Can you work these out from the model? Positions are in its coordinate system, mm. Give positions to 0.01 mm unless a question says otherwise; leave off trailing zeros. Loops run counter-clockwise (first coordinate to the right, second up) from the corner with the lowest first, then second, coordinate; pieces in that order, holes last. Notation, with made-up numbers: (53.25, 10.5) - (86.25, 10.5) arc R22 cw to (86.25, 35.5) - close; hole circle Ø6 at (-12.5, 45.25). An arc over 180 degrees is marked (long way). Answer in a Markdown table with one row per item.
from build123d import *

# Parameters (mm, degrees)
BOSS_EXTRUDE1_DEPTH = 0.05
FILLET1_R           = 1


with BuildPart() as part:
    # frame_outline → Boss-Extrude1 (new, symmetric)
    with BuildSketch(Plane.XY):
        Polygon((0, 0), (3, 0), (3, -0.25), (4, -0.25), (4, 0), (4.5, 0), (5.266044443, 0.64278761), (5.426741346, 0.451276499), (6.192785789, 1.094064109), (6.032088886, 1.285575219), (6.606622219, 1.767665927), (5.050898392, 1.767665927), (4.136029766, 1), (-4.136029766, 1), (-5.050898392, 1.767665927), (-6.606622219, 1.767665927), (-6.032088886, 1.285575219), (-6.192785789, 1.094064109), (-5.426741346, 0.451276499), (-5.266044443, 0.64278761), (-4.5, 0), (-4, 0), (-4, -0.25), (-3, -0.25), (-3, 0), align=None)
    extrude(amount=BOSS_EXTRUDE1_DEPTH, both=True)

    # Fillet1
    fillet1_edges = [part.edges().sort_by_distance(p)[0] for p in [
        (-5.050898392, 1.767665927, 0),
        (-4.136029766, 1, 0),
        (4.136029766, 1, 0),
        (5.050898392, 1.767665927, 0),
    ]]
    fillet(fillet1_edges, radius=FILLET1_R)


solid = part.part
Q1. If I drill on line 1 (X direction, y = 1.4, z = 0); line 2 (X direction, y = 1.55, z = 0); line 3 (Y direction, x = 3.5, z = 0), over which ranges is the centre line in solid material (lowest first)? Write a range as [from, to].
Checked values:
| item | result |
|---|---|
| line 1 | x = [-6.17, -4.61], [4.61, 6.17] |
| line 2 | x = [-6.35, -4.79], [4.79, 6.35] |
| line 3 | y = [-0.25, 1] |
Q2. Imagine slicing it at B-B, the plane x = -0.75. Write out the boundary of the cut face in (y, z).
Checked values:
| item | result |
|---|---|
| outline | (0, -0.05) - (1, -0.05) - (1, 0.05) - (0, 0.05) - close |
Q3. Imagine slicing it at A-A, the plane z = 0. Write out the boundary of the cut face in (x, y), and give its area (3 significant figures).
Checked values:
| item | result |
|---|---|
| outline | (-6.61, 1.77) - (-6.03, 1.29) - (-6.19, 1.09) - (-5.43, 0.45) - (-5.27, 0.64) - (-4.5, 0) - (-4, 0) - (-4, -0.25) - (-3, -0.25) - (-3, 0) - (3, 0) - (3, -0.25) - (4, -0.25) - (4, 0) - (4.5, 0) - (5.27, 0.64) - (5.43, 0.45) - (6.19, 1.09) - (6.03, 1.29) - (6.61, 1.77) - (5.41, 1.77) arc R1 ccw to (4.77, 1.53) - (4.41, 1.23) arc R1 cw to (3.77, 1) - (-3.77, 1) arc R1 cw to (-4.41, 1.23) - (-4.77, 1.53) arc R1 ccw to (-5.41, 1.77) - close |
| area | 13.6 mm² |
Q4. Imagine slicing it at C-C, the plane y = 0.15. Write out the boundary of the cut face in (x, z).
Checked values:
| item | result |
|---|---|
| outline | (-4.68, -0.05) - (4.68, -0.05) - (4.68, 0.05) - (-4.68, 0.05) - close |
